Can you work these out from the model? Positions are in its coordinate system, mm. Face numbers are marked on the shaded views. A direction names the side the tool comes from. Coordinates: 2 decimals unless noted, no trailing zeros. Write each loop counter-clockwise with the first axis right and the second up, starting at its lowest first coordinate (ties: lowest second). Pieces come first, ordered by that corner, then holes. Notation, with made-up numbers: (2.5, 63) - (52.5, 63) arc R31 cw to (52.5, 93) - close; hole circle Ø4 at (3, 53). An arc over 180 degrees is marked (long way). One line per question, with ' | ' between items. Start each with the question number.
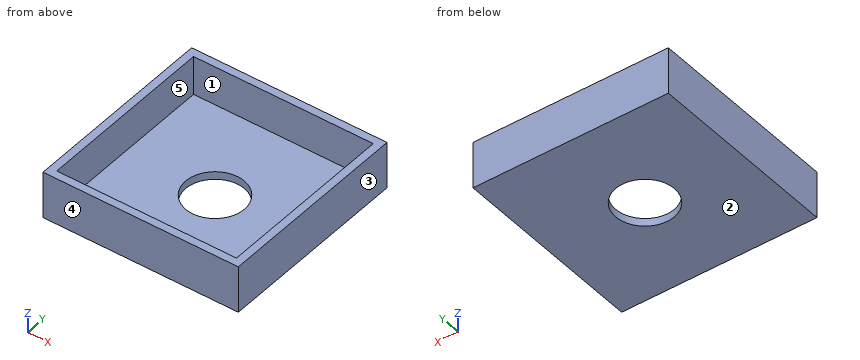
from build123d import *

# Parameters (mm, degrees)
F0_W     = 50
F0_H     = 50
F0_R     = 7.5
F2_DEPTH = 2
F1_W     = 50
F1_H     = 50
F1_W_2   = 46
F1_H_2   = 46
F3_DEPTH = 10


with BuildPart() as f2:
    # F0 (on Top) → F2 (new body)
    with BuildSketch(Plane.XY):
        Rectangle(F0_W, F0_H)
        Circle(F0_R, mode=Mode.SUBTRACT)
    extrude(amount=-F2_DEPTH)

    # F1 (on face) → F3 (join)
    with BuildSketch(Plane.XY):
        Rectangle(F1_W, F1_H)
        Rectangle(F1_W_2, F1_H_2, mode=Mode.SUBTRACT)
    extrude(amount=F3_DEPTH)


solid = f2.part
(1) If we section it at A-A on y = 0: List the corners of the cut face in (x, z) for me, plus the area to 3 significant figures.
(2) If we mould it in two halves opening along Y, with no side actions, what happens to the marked faces 3, 4 and 5? For each: +Y half, -Y half, draft (parallel to the pull), parting line (faces both ways), or undercut.
(3) If I drill on probe 1 along X at (y, z) = (-8, 2.25); probe 2 along Y at (x, z) = (0, -0.4), over which ranges is the centre line in solid material (lowest first)?
(4) If we section it at C-C on z = 2.75: List the corners of the cut face in (x, y) for me, plus the area to 3 significant figures.
(5) If we section it at D-D on y = 20: List the corners of the cut face in (x, z) for me, plus the area to 3 significant figures.
(6) Which directions (+Z, -Z, +X, -X, +Y, -Y) give clear straight access to the entire face, cutting with the end or side of a thin tool? Please do the marked faces 1 and 2.
(7) I'm going to push a flat-ended pin straight in: pin 1 (8 mm diameter, centred on x = 7, y = 15, fed in from +Z). Where does the tip first touch, or does it pass through?
Values:
1) outline: (-25, -2) - (-7.5, -2) - (-7.5, 0) - (-23, 0) - (-23, 10) - (-25, 10) - close; (7.5, -2) - (25, -2) - (25, 10) - (23, 10) - (23, 0) - (7.5, 0) - close | area: 110 mm2
2) face 3: draft | face 4: -Y half | face 5: undercut
3) probe 1: -25 to -23, 23 to 25 | probe 2: -25 to -7.5, 7.5 to 25
4) outline: (-25, -25) - (25, -25) - (25, 25) - (-25, 25) - close; hole (-23, -23) - (23, -23) - (23, 23) - (-23, 23) - close | area: 384 mm2
5) outline: (-25, -2) - (25, -2) - (25, 10) - (23, 10) - (23, 0) - (-23, 0) - (-23, 10) - (-25, 10) - close | area: 140 mm2
6) face 1: +Z | face 2: -Z, +X, -X, +Y, -Y
7) pin 1: z = 0
